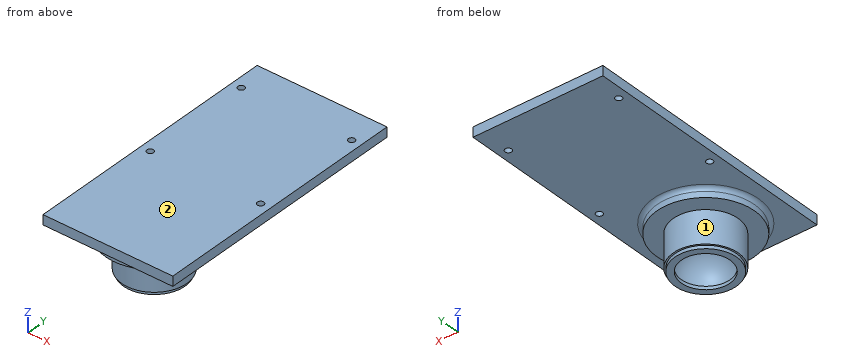
from build123d import *

# Parameters (mm, degrees)
SKETCH1_W           = 40
SKETCH1_H           = 80
BOSS_EXTRUDE1_DEPTH = 3
SKETCH2_R           = 1
CUT_EXTRUDE1_DEPTH  = 3
SKETCH3_R           = 15
BOSS_EXTRUDE2_DEPTH = 3
FILLET1_R           = 1.2
SKETCH4_R           = 10
BOSS_EXTRUDE3_DEPTH = 10
SKETCH14_R          = 9.5
BOSS_EXTRUDE4_DEPTH = 1
SKETCH15_R          = 7.5
CUT_EXTRUDE7_DEPTH  = 1


with BuildPart() as part:
    # Sketch1 → Boss-Extrude1 (new body)
    with BuildSketch(Plane.XY):
        with Locations((20, 40)):
            Rectangle(SKETCH1_W, SKETCH1_H)
    extrude(amount=BOSS_EXTRUDE1_DEPTH)

    # Sketch2 → Cut-Extrude1 (cut)
    with BuildSketch(Plane.XY.offset(3)):
        with Locations((3, 70.446149139)):
            Circle(SKETCH2_R)
        with Locations((3, 36.446149139)):
            Circle(SKETCH2_R)
        with Locations((37, 70.446149139)):
            Circle(SKETCH2_R)
        with Locations((37, 36.446149139)):
            Circle(SKETCH2_R)
    extrude(amount=-CUT_EXTRUDE1_DEPTH, mode=Mode.SUBTRACT)

    # Sketch3 → Boss-Extrude2 (add)
    with BuildSketch(Plane(origin=(0, 0, 0), x_dir=(-1, 0, 0), z_dir=(0, 0, -1))):
        with Locations((-20, 17.303489874)):
            Circle(SKETCH3_R)
    extrude(amount=BOSS_EXTRUDE2_DEPTH)

    # Fillet1
    fillet1_edges = [part.edges().sort_by_distance(p)[0] for p in [
        (35, 17.303489874, 0),
    ]]
    fillet(fillet1_edges, radius=FILLET1_R)

    # Sketch4 → Boss-Extrude3 (add)
    with BuildSketch(Plane(origin=(0, 0, -3), x_dir=(-1, 0, 0), z_dir=(0, 0, -1))):
        with Locations((-20, 17.303489874)):
            Circle(SKETCH4_R)
    extrude(amount=BOSS_EXTRUDE3_DEPTH)

    # Sketch10 → Cut-Revolve2 (revolve, cut)
    with BuildSketch(Plane(origin=(0, 0, -13), x_dir=(-1, 0, 0), z_dir=(0, 0, -1))):
        with BuildLine():
            Line((-20, 25.837066369), (-20, 8.769913378))
            ThreePointArc((-20, 8.769913378), (-11.466423505, 17.303489874), (-20, 25.837066369))
        make_face()
    revolve(axis=Axis((20, 25.837066369, -13), (0, -1, 0)), mode=Mode.SUBTRACT)

    # Sketch14 → Boss-Extrude4 (add)
    with BuildSketch(Plane(origin=(0, 0, -13), x_dir=(-1, 0, 0), z_dir=(0, 0, -1))):
        with Locations((-20, 17.303489874)):
            Circle(SKETCH14_R)
    extrude(amount=BOSS_EXTRUDE4_DEPTH)

    # Sketch15 → Cut-Extrude7 (cut)
    with BuildSketch(Plane(origin=(0, 0, -14), x_dir=(-1, 0, 0), z_dir=(0, 0, -1))):
        with Locations((-20, 17.303489874)):
            Circle(SKETCH15_R)
    extrude(amount=-CUT_EXTRUDE7_DEPTH, mode=Mode.SUBTRACT)


solid = part.part
Geometry: final body of the model. Coordinates: model frame, mm. Face numbers are marked on the shaded views. A direction names the side the tool comes from. Coordinates: 2 decimals unless noted, no trailing zeros. Write each loop counter-clockwise with the first axis right and the second up, starting at its lowest first coordinate (ties: lowest second). Pieces come first, ordered by that corner, then holes. Notation, with made-up numbers: (42, 28) - (75, 28) arc R16 cw to (75, 47) - close; hole circle Ø6 at (45, -19.5). An arc over 180 degrees is marked (long way). Return JSON: item names as keys, results as strings.
Item 1: Section query C-C (y = 64). Output: boundary loops of the cut face in (x, z), and give its area (3 significant figures).
Completed:
{"outline": "(0, 0) - (40, 0) - (40, 3) - (0, 3) - close", "area": "120 mm2"}
Item 2: Reachability of the marked faces 1 and 2 from +Z, -Z, +X, -X, +Y, -Y: full face, straight path, thin tool, end or side. Return the list, or none.
Completed:
{"face 1": "-Z", "face 2": "+Z, +X, -X, +Y, -Y"}
Item 3: Section query A-A (x = 3). Output: boundary loops of the cut face in (y, z).
Completed:
{"outline": "(0, 0) - (35.45, 0) - (35.45, 3) - (0, 3) - close; (37.45, 0) - (69.45, 0) - (69.45, 3) - (37.45, 3) - close; (71.45, 0) - (80, 0) - (80, 3) - (71.45, 3) - close"}
Item 4: Line query: L1, parallel to Y at x = 37, z = 1.1; L2, parallel to X at y = 70, z = 1; L3, parallel to Y at x = 20, z = -13.55. Output: solid intervals per line, ascending.
Completed:
{"L1": "y = 0 to 35.45, 37.45 to 69.45, 71.45 to 80", "L2": "x = 0 to 2.11, 3.89 to 36.11, 37.89 to 40", "L3": "y = 7.8 to 9.8, 24.8 to 26.8"}
Item 5: Pin query (flat end, axial travel): pin 1 Ø10 at (x, z) = (11, -12) entering from +Y; pin 2 Ø12 at (x, y) = (20.5, 49) entering from -Z; pin 3 Ø1 at (x, z) = (33, -3) entering from +Y. Return the tip coordinate at first contact, or that it passes through.
Completed:
{"pin 1": "stops at y = 26.47", "pin 2": "stops at z = 0", "pin 3": "stops at y = 25.6"}
Item 6: Section query D-D (z = -7.5). Output: boundary loops of the cut face in (x, y).
Completed:
{"outline": "circle Ø20 at (20, 17.3); hole circle Ø13.05 at (20, 17.3)"}
Item 7: Section query B-B (x = 20). Output: boundary loops of the cut face in (y, z), and give its area (3 significant figures).
Completed:
{"outline": "(0, 0) - (1.1, 0) arc R1.2 cw to (2.3, -1.2) - (2.3, -3) - (7.3, -3) - (7.3, -13) - (7.8, -13) - (7.8, -14) - (9.8, -14) - (9.8, -13) - (8.77, -13) arc R8.53 cw to (25.84, -13) - (24.8, -13) - (24.8, -14) - (26.8, -14) - (26.8, -13) - (27.3, -13) - (27.3, -3) - (32.3, -3) - (32.3, -1.2) arc R1.2 cw to (33.5, 0) - (80, 0) - (80, 3) - (0, 3) - close", "area": "420 mm2"}
